Input: dimensioned drawing with shaded views. Units: mm. Origin: part minimum x, y, z. Coordinates: 2 decimals unless noted, no trailing zeros. Order: outer loops, then holes, each group sorted by start corner. A loop starts at its lowest first (then second) coordinate and runs counter-clockwise, first axis right, second up. Notation, with made-up numbers: (6.5, 42) - (20.5, 42) arc R20 ccw to (20.5, 63) - close; hole circle Ø8 at (-31.5, 25). An arc over 180 degrees is marked (long way). Use one line per item in the form item = value. Start each with the question number.
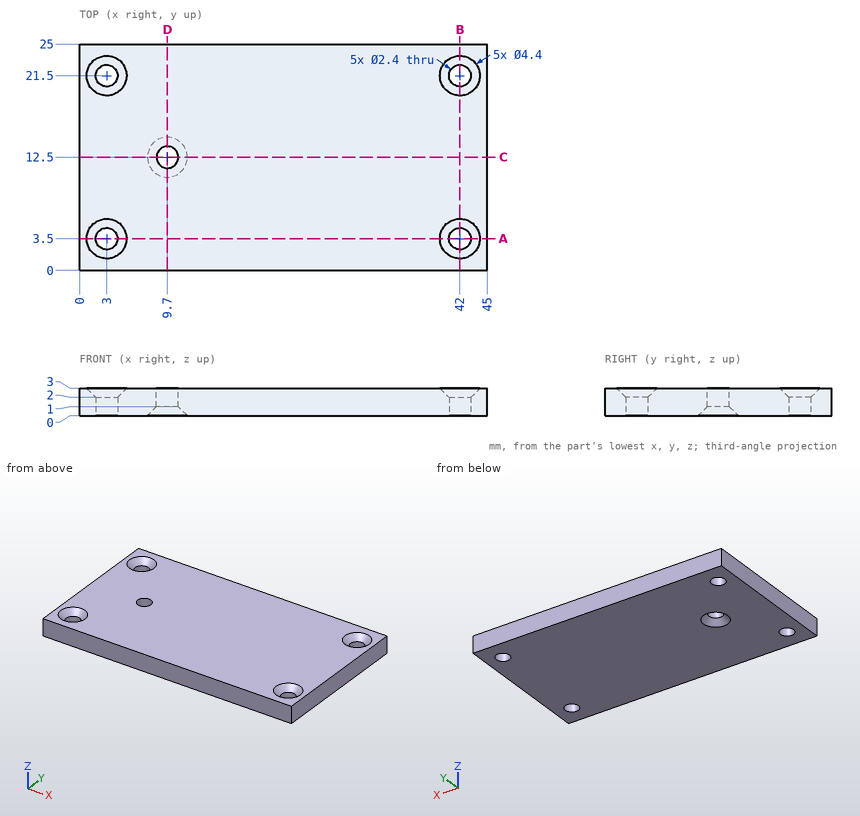
(1) Cut plane B-B on x = 42. Return the cut outline in (y, z).
(2) Cut plane A-A on y = 3.5. Return the cut outline in (x, z), plus the area to 3 significant figures.
(3) Cut plane D-D on x = 9.7. Return the cut outline in (y, z).
(4) Cut plane C-C on y = 12.5. Return the cut outline in (x, z).
(5) Material intervals for L1, parallel to X at y = 3.5, z = 0.7; L2, parallel to Y at x = 3, z = 1.35; L3, parallel to X at y = 22.5, z = 0.2, sorted ascending. Write a range as from..to.
(6) Contact query for flat-ended pins moving along their axis: pin 1 Ø2 at (x, y) = (9.7, 12.5) entering from -Z; pin 2 Ø3 at (x, y) = (42, 21.5) entering from +Z. Output: stop coordinate, or through.
Check sheet entries:
q1.outline = (0, 0) - (2.3, 0) - (2.3, 2) - (1.3, 3) - (0, 3) - close; (4.7, 0) - (20.3, 0) - (20.3, 2) - (19.3, 3) - (5.7, 3) - (4.7, 2) - close; (22.7, 0) - (25, 0) - (25, 3) - (23.7, 3) - (22.7, 2) - close
q2.outline = (0, 0) - (1.8, 0) - (1.8, 2) - (0.8, 3) - (0, 3) - close; (4.2, 0) - (40.8, 0) - (40.8, 2) - (39.8, 3) - (5.2, 3) - (4.2, 2) - close; (43.2, 0) - (45, 0) - (45, 3) - (44.2, 3) - (43.2, 2) - close
q2.area = 119 mm^2
q3.outline = (0, 0) - (10.3, 0) - (11.3, 1) - (11.3, 3) - (0, 3) - close; (13.7, 1) - (14.7, 0) - (25, 0) - (25, 3) - (13.7, 3) - close
q4.outline = (0, 0) - (7.5, 0) - (8.5, 1) - (8.5, 3) - (0, 3) - close; (10.9, 1) - (11.9, 0) - (45, 0) - (45, 3) - (10.9, 3) - close
q5.L1 = 0..1.8, 4.2..40.8, 43.2..45
q5.L2 = 0..2.3, 4.7..20.3, 22.7..25
q5.L3 = 0..2.34, 3.66..41.34, 42.66..45
q6.pin_1 = through
q6.pin_2 = 2.3
